Here's the drawing with two shaded views (mm, measured from the low corner). I have some questions. Round coordinates to 2 decimals unless told otherwise and drop trailing zeros. Write each loop counter-clockwise with the first axis right and the second up, starting at its lowest first coordinate (ties: lowest second). Pieces come first, ordered by that corner, then holes. Notation, with made-up numbers: M 50,33 L 96,33 A25 ccw 96,54 Z; hole C 60.25,79.5 d10. An arc over 180 degrees is marked long. Write item = value, one per line. Start each with the question number.
(1) Will this pin go through, and if not, where does the flat tip stop? pin 1 Ø3 at (x, z) = (5, 4.5) entering from -Y.
(2) I need wall thicknesses on line 1 along Z through (x, y) = (195, 1.6); line 2 along Z through (x, y) = (151.5, 3.9) (1 decimal). Which ranges of each line are inside material? Lowest first, please.
(3) I want a section at B-B (x = 195). List the corners of the cut face in (y, z) for me, and give its area (3 significant figures).
(4) I want a section at A-A (y = 3.45). Give the number of separate pieces and of enclosed holes in the cut face, and give its area (3 significant figures).
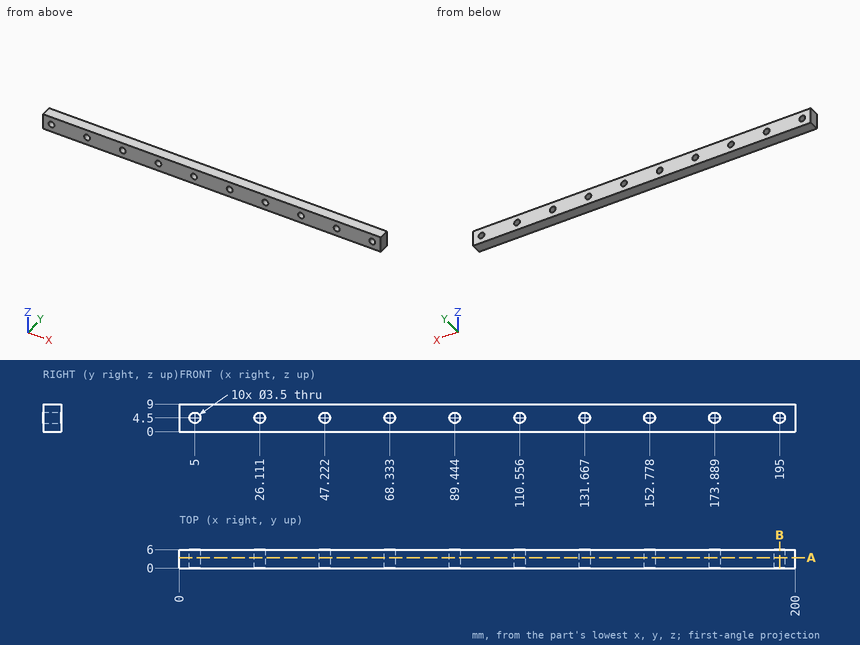
Returned:
q1.pin_1 = through
q2.line_1 = 0 to 2.75, 6.25 to 9
q2.line_2 = 0 to 3.3, 5.7 to 9
q3.outline = M 0,0 L 6,0 L 6,2.75 L 0,2.75 Z; M 0,6.25 L 6,6.25 L 6,9 L 0,9 Z
q3.area = 33.0 mm²
q4.separate_pieces = 1
q4.enclosed_holes = 10
q4.area = 1,700 mm²
